```python
from build123d import *

# Parameters (mm, degrees)
SKETCH1_R           = 10.89504564
BOSS_EXTRUDE1_DEPTH = 38.1
SKETCH2_W           = 22.352
SKETCH2_H           = 19.05
BOSS_EXTRUDE2_DEPTH = 2.44693827
SKETCH3_W           = 63.5
SKETCH3_H           = 8.943070636
BOSS_EXTRUDE3_DEPTH = 63.5
BOSS_EXTRUDE4_DEPTH = 63.5


with BuildPart() as part:
    # Sketch1 → Boss-Extrude1 (new body)
    with BuildSketch(Plane.XY):
        Circle(SKETCH1_R)
    extrude(amount=-BOSS_EXTRUDE1_DEPTH)

    # Sketch2 → Boss-Extrude2 (add)
    with BuildSketch(Plane(origin=(0, 0, -38.1), x_dir=(-1, 0, 0), z_dir=(0, 0, -1))):
        with Locations((0, 9.525)):
            Rectangle(SKETCH2_W, SKETCH2_H)
    extrude(amount=-BOSS_EXTRUDE2_DEPTH)

    # Sketch3 → Boss-Extrude3 (add)
    with BuildSketch(Plane(origin=(0, 0, -38.1), x_dir=(-1, 0, 0), z_dir=(0, 0, -1))):
        with Locations((0, 23.521535318)):
            Rectangle(SKETCH3_W, SKETCH3_H)
    extrude(amount=-BOSS_EXTRUDE3_DEPTH)

    # Sketch4 → Boss-Extrude4 (add)
    with BuildSketch(Plane(origin=(0, 0, -38.1), x_dir=(-1, 0, 0), z_dir=(0, 0, -1))):
        Polygon((-31.75, 27.993070636), (-31.75, 66.093070636), (-6.35, 66.093070636), (-6.35, 86.090384505), (-38.747245179, 86.090384505), (-38.747245179, 19.05), (-31.75, 19.05), align=None)
        Polygon((31.75, 27.993070636), (31.75, 66.093070636), (6.35, 66.093070636), (6.35, 86.090384505), (38.747245179, 86.090384505), (38.747245179, 19.05), (31.75, 19.05), align=None)
    extrude(amount=-BOSS_EXTRUDE4_DEPTH)


solid = part.part
```
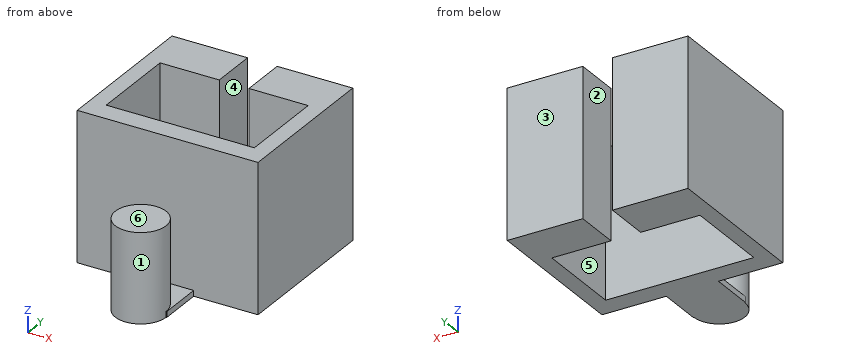
Build history of the part. All positions in model axes, mm. Face numbers are marked on the shaded views. A direction names the side the tool comes from. Round coordinates to 2 decimals unless told otherwise and drop trailing zeros. Write each loop counter-clockwise with the first axis right and the second up, starting at its lowest first coordinate (ties: lowest second). Pieces come first, ordered by that corner, then holes. Notation, with made-up numbers: (-4, 67.25) -> (20, 67.25) arc R20 cw to (20, 92.25) -> close; hole circle Ø3 at (14.25, -36.75). An arc over 180 degrees is marked (long way). Put each result on its own line as item: value.
Item 1: Slice it at B-B, the plane y = 45. Give the cut face in (x, z), plus the area to 3 significant figures.
Here are the results:
outline: (-38.75, -38.1) -> (-31.75, -38.1) -> (-31.75, 25.4) -> (-38.75, 25.4) -> close; (31.75, -38.1) -> (38.75, -38.1) -> (38.75, 25.4) -> (31.75, 25.4) -> close
area: 889 mm^2
Item 2: Slice it at D-D, the plane z = 4. Give the cut face in (x, y).
Here are the results:
outline: (-38.75, 19.05) -> (38.75, 19.05) -> (38.75, 86.09) -> (6.35, 86.09) -> (6.35, 66.09) -> (31.75, 66.09) -> (31.75, 27.99) -> (-31.75, 27.99) -> (-31.75, 66.09) -> (-6.35, 66.09) -> (-6.35, 86.09) -> (-38.75, 86.09) -> close
Item 3: Wall check: probe 1 along X at (y, z) = (64.5, -15); probe 2 along Y at (x, z) = (-20, -22); probe 3 along X at (y, z) = (69, 6.5). Give the ranges that are in metal, low to high. Write a range as from..to.
Here are the results:
probe 1: x = -38.75..-31.75, 31.75..38.75
probe 2: y = 19.05..27.99, 66.09..86.09
probe 3: x = -38.75..-6.35, 6.35..38.75
Item 4: Tool access for the marked faces 4, 5 and 6: list every direction of +Z, -Z, +X, -X, +Y, -Y with a clear straight run to the whole face (end or side of a thin tool).
Here are the results:
face 4: +Z, -Z, +Y
face 5: +Z, -Z
face 6: +Z, +X, -X, -Y
Item 5: Flat gauge pins, fed straight in: P1, Ø2.5, axis at y = 5.5, z = -37.5, coming from the -X side; P2, Ø12, axis at x = 12, z = 17.5, coming from the -Y side; P3, Ø9.5, axis at x = -1.5, y = 11, coming from the +Z side. Where does each tip first touch, or does it go through?
Here are the results:
P1: stops at x = -11.18
P2: stops at y = 19.05
P3: stops at z = 0
Item 6: Two-plate mould, pull along Y, no slides. Class the marked faces 1, 2 and 3: pulls with the +Y half, pulls with the -Y half, needs draft (parallel to the pull), parting line crosses it, or undercut.
Here are the results:
face 1: undercut
face 2: needs draft
face 3: pulls with the +Y half
Item 7: Slice it at C-C, the plane x = 18. Give the cut face in (y, z).
Here are the results:
outline: (19.05, -38.1) -> (27.99, -38.1) -> (27.99, 25.4) -> (19.05, 25.4) -> close; (66.09, -38.1) -> (86.09, -38.1) -> (86.09, 25.4) -> (66.09, 25.4) -> close
Item 8: Slice it at A-A, the plane z = -3. Give the cut face in (x, y).
Here are the results:
outline: (-38.75, 19.05) -> (38.75, 19.05) -> (38.75, 86.09) -> (6.35, 86.09) -> (6.35, 66.09) -> (31.75, 66.09) -> (31.75, 27.99) -> (-31.75, 27.99) -> (-31.75, 66.09) -> (-6.35, 66.09) -> (-6.35, 86.09) -> (-38.75, 86.09) -> close; circle Ø21.79 at (0, 0)
